Geometry: final body of the model. Coordinates: model frame, mm. A direction names the side the tool comes from. Coordinates: 2 decimals unless noted, no trailing zeros. Loops run counter-clockwise (first coordinate to the right, second up) from the corner with the lowest first, then second, coordinate; pieces in that order, holes last. Notation, with made-up numbers: (-26, -13.5) - (-7, -13.5) arc R12 cw to (-7, 8.5) - close; hole circle Ø10 at (61, -17). An arc over 180 degrees is marked (long way). Put each result on its own line as item: value. Start each with the question number.
1) Section B-B on z = -34.5. Output: boundary loops of the cut face in (x, y), and give its area (3 significant figures).
2) Draft query along X for faces 1 (the cylindrical face through (224.78, -3.22, 72.58)), 2 (the flat face through (77, -3, 50.8)), 3 (the flat face through (78, -6.35, 52)). Return one class per face: +X half, -X half, draft (parallel to the pull), parting line (faces both ways), or undercut.
3) Section C-C on z = 19.5. Output: boundary loops of the cut face in (x, y), and give its area (3 significant figures).
4) Material intervals for line 1 along Z through (x, y) = (97.5, -5); line 2 along X through (y, z) = (-0.5, -18); line 3 along X through (y, z) = (-3.5, 34.5), sorted ascending. Write a range as from..to.
5) Contact query for a flat-ended pin moving along its axis: pin 1 Ø1.9 at (x, y) = (74, -3) entering from -Z. Output: stop coordinate, or through.
6) Reachability of faces 4 (the flat face through (3.84, -3.13, -13.49)), 5 (the flat face through (-76.2, -3, 1)) from +Z, -Z, +X, -X, +Y, -Y: full face, straight path, thin tool, end or side. Return the list, or none.
7) Section D-D on x = 49.5. Output: boundary loops of the cut face in (y, z).
8) Section A-A on y = -3.5. Output: boundary loops of the cut face in (x, z), and give its area (3 significant figures).
```python
from build123d import *

# Parameters (mm, degrees)
F1_DEPTH = 6.35
F3_R     = 12.7


with BuildPart() as f1:
    # F0 (on Front) → F1 (new body)
    with BuildSketch(Plane.XZ):
        Polygon((76.2, 76.2), (-76.2, 76.2), (-76.2, -76.2), (-25.4, -76.2), (33.8210725857, 50.8), (76.2, 50.8), align=None)
    extrude(amount=F1_DEPTH)

    # F2: F1 across face


with BuildPart() as f1_1:
    add(f1.part)
    add(f1.part.mirror(Plane(origin=(76.2, -3.175, 63.5), x_dir=(0, 1, 0), z_dir=(1, 0, 0))))

    # F3
    f3_edges = [f1_1.edges().sort_by_distance(p)[0] for p in [
        (33.821073, -3.175, 50.8),
        (118.578927, -3.175, 50.8),
        (177.8, -3.175, -76.2),
        (-25.4, -3.175, -76.2),
        (-76.2, -3.175, -76.2),
        (228.6, -3.175, -76.2),
        (228.6, -3.175, 76.2),
        (-76.2, -3.175, 76.2),
    ]]
    fillet(f3_edges, radius=F3_R)


solid = f1_1.part
```
Answer block:
1. outline: (-76.2, -6.35) - (-5.95, -6.35) - (-5.95, 0) - (-76.2, 0) - close; (158.35, -6.35) - (228.6, -6.35) - (228.6, 0) - (158.35, 0) - close
1. area: 892 mm²
2. face 1: +X half
2. face 2: undercut
2. face 3: draft
3. outline: (-76.2, -6.35) - (19.23, -6.35) - (19.23, 0) - (-76.2, 0) - close; (133.17, -6.35) - (228.6, -6.35) - (228.6, 0) - (133.17, 0) - close
3. area: 1,210 mm²
4. line 1: z = 50.8..76.2
4. line 2: x = -76.2..1.74, 150.66..228.6
4. line 3: x = -76.2..26.22, 126.18..228.6
5. pin 1: stops at z = 50.8
6. face 4: -Z, +Y, -Y
6. face 5: +Z, -Z, -X, +Y, -Y
7. outline: (-6.35, 50.8) - (0, 50.8) - (0, 76.2) - (-6.35, 76.2) - close
8. outline: (-76.2, -63.5) arc R12.7 ccw to (-63.5, -76.2) - (-33.49, -76.2) arc R12.7 ccw to (-21.98, -68.87) - (30.4, 43.47) arc R12.7 cw to (41.91, 50.8) - (110.49, 50.8) arc R12.7 cw to (122, 43.47) - (174.38, -68.87) arc R12.7 ccw to (185.89, -76.2) - (215.9, -76.2) arc R12.7 ccw to (228.6, -63.5) - (228.6, 63.5) arc R12.7 ccw to (215.9, 76.2) - (-63.5, 76.2) arc R12.7 ccw to (-76.2, 63.5) - close
8. area: 28,000 mm²
